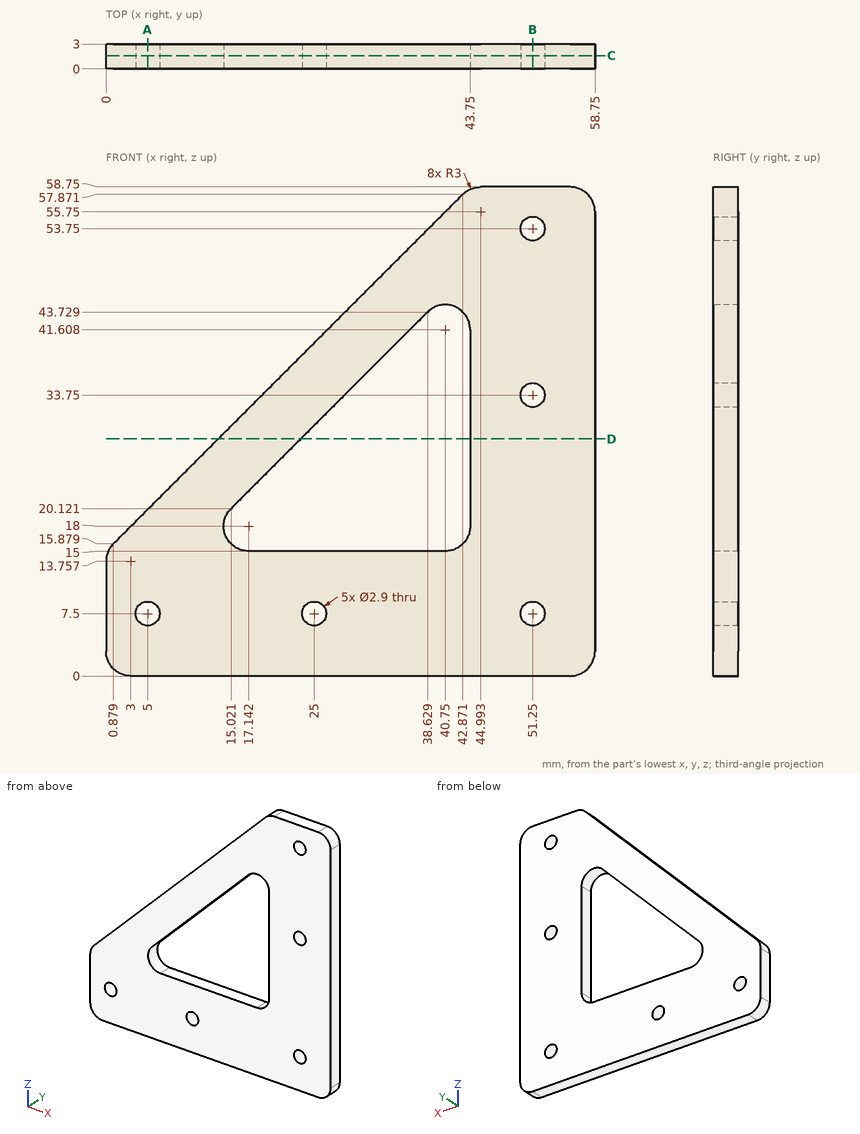
Drawing for the job (mm, zero at the part's lowest x, y, z). Give positions to 0.01 mm unless a question says otherwise; leave off trailing zeros. Order: outer loops, then holes, each group sorted by start corner. A loop starts at its lowest first (then second) coordinate and runs counter-clockwise, first axis right, second up. Notation, with made-up numbers: (5, 39.5) -> (22, 39.5) arc R30 cw to (22, 75.5) -> close; hole circle Ø4 at (49.5, 50). An arc over 180 degrees is marked (long way). Use one line per item in the form item = value.
(1) Drill centre lines: line 1 (X direction, y = 1.4, z = 7.5); line 2 (X direction, y = 2.05, z = 38); line 3 (Z direction, x = 22.5, y = 1.15). Where is each one in solid material? Low to high. Write a range as from..to.
Solution:
line_1 = 0..3.55, 6.45..23.55, 26.45..49.8, 52.7..58.75
line_2 = 23..32.9, 43.75..58.75
line_3 = 0..15, 27.6..37.5
(2) Saw through at A-A (x = 5). Write the cut outline in (y, z).
Solution:
outline = (0, 0) -> (3, 0) -> (3, 6.05) -> (0, 6.05) -> close; (0, 8.95) -> (3, 8.95) -> (3, 20) -> (0, 20) -> close
(3) Saw through at C-C (y = 1.6). Write the cut outline in (x, z), then the cut area to 3 significant figures.
Solution:
outline = (0, 3) arc R3 ccw to (3, 0) -> (55.75, 0) arc R3 ccw to (58.75, 3) -> (58.75, 55.75) arc R3 ccw to (55.75, 58.75) -> (44.99, 58.75) arc R3 ccw to (42.87, 57.87) -> (0.88, 15.88) arc R3 ccw to (0, 13.76) -> close; hole circle Ø2.9 at (5, 7.5); hole (15.02, 20.12) arc R3 ccw to (17.14, 15) -> (40.75, 15) arc R3 ccw to (43.75, 18) -> (43.75, 41.61) arc R3 ccw to (38.63, 43.73) -> close; hole circle Ø2.9 at (25, 7.5); hole circle Ø2.9 at (51.25, 7.5); hole circle Ø2.9 at (51.25, 33.75); hole circle Ø2.9 at (51.25, 53.75)
area = 1,910 mm²
(4) Saw through at B-B (x = 51.25). Write the cut outline in (y, z).
Solution:
outline = (0, 0) -> (3, 0) -> (3, 6.05) -> (0, 6.05) -> close; (0, 8.95) -> (3, 8.95) -> (3, 32.3) -> (0, 32.3) -> close; (0, 35.2) -> (3, 35.2) -> (3, 52.3) -> (0, 52.3) -> close; (0, 55.2) -> (3, 55.2) -> (3, 58.75) -> (0, 58.75) -> close
(5) Saw through at D-D (z = 28.5). Write the cut outline in (x, y).
Solution:
outline = (13.5, 0) -> (23.4, 0) -> (23.4, 3) -> (13.5, 3) -> close; (43.75, 0) -> (58.75, 0) -> (58.75, 3) -> (43.75, 3) -> close
